from build123d import *

# Parameters (mm, degrees)
SKETCH_1_R      = 6.1
EXTRUDE_1_DEPTH = 4


with BuildPart() as part:
    # 스케치1 → 보스-돌출1 (new body)
    with BuildSketch(Plane.XY):
        with BuildLine():
            Line((-10.9, 20.333989173), (-10.9, 2.333989173))
            Line((-10.9, 2.333989173), (-8.65, 2.333989173))
            Line((-8.65, 2.333989173), (8.65, 2.333989173))
            Line((8.65, 2.333989173), (10.9, 2.333989173))
            Line((10.9, 2.333989173), (10.9, 20.333989173))
            ThreePointArc((10.9, 20.333989173), (0, 31.233989173), (-10.9, 20.333989173))
        make_face()
        with Locations((0, 20.333989173)):
            Circle(SKETCH_1_R, mode=Mode.SUBTRACT)
    extrude(amount=EXTRUDE_1_DEPTH)


solid = part.part
Model file for the job. Use its own axes, mm. Round coordinates to 2 decimals unless told otherwise and drop trailing zeros. Order: outer loops, then holes, each group sorted by start corner. A loop starts at its lowest first (then second) coordinate and runs counter-clockwise, first axis right, second up.
(1) Pin check, flat tip, straight feed: pin 1 (12 mm diameter, centred on x = -0.5, y = 9.5, fed in from -Z). Stop position of the tip, or through.
(2) Band-saw the part on A-A (y = 23.5). List the corners of the cut face in (x, z).
(3) Drill centre lines: line 1 (Y direction, x = 0, z = 1.1); line 2 (Y direction, x = -1.25, z = 1.95); line 3 (X direction, y = 21.25, z = 0.65). Where is each one in solid material? Low to high.
(4) Band-saw the part on C-C (z = 2.25). List the corners of the cut face in (x, y), then the cut area to 3 significant figures.
(5) Pull direction X, two halves, no side cores. Call faces 1 (the face through (-4.84, 16.62, 1.97)), 2 (the face through (0, 2.334, 2)), 3 (the face through (-10.9, 11, 2)): released by +X, released by -X, zero draft, split by the parting line, or undercut.
(6) Band-saw the part on B-B (x = 0). List the corners of the cut face in (y, z).
(7) Band-saw the part on D-D (x = -6.5). List the corners of the cut face in (y, z).
Verdict:
1. pin 1: stops at z = 0
2. outline: (-10.43, 0) - (-5.21, 0) - (-5.21, 4) - (-10.43, 4) - close; (5.21, 0) - (10.43, 0) - (10.43, 4) - (5.21, 4) - close
3. line 1: y = 2.33 to 14.23, 26.43 to 31.23
3. line 2: y = 2.33 to 14.36, 26.3 to 31.16
3. line 3: x = -10.86 to -6.03, 6.03 to 10.86
4. outline: (-10.9, 2.33) - (10.9, 2.33) - (10.9, 20.33) arc R10.9 ccw to (-10.9, 20.33) - close; hole circle Ø12.2 at (0, 20.33)
4. area: 462 mm2
5. face 1: undercut
5. face 2: zero draft
5. face 3: released by -X
6. outline: (2.33, 0) - (14.23, 0) - (14.23, 4) - (2.33, 4) - close; (26.43, 0) - (31.23, 0) - (31.23, 4) - (26.43, 4) - close
7. outline: (2.33, 0) - (29.08, 0) - (29.08, 4) - (2.33, 4) - close
